```python
from build123d import *

# Parameters (mm, degrees)
F1_DEPTH = 33.02
F0_R     = 2.6264362
F0_R_2   = 2.6264304873
F2_DEPTH = 38.1


with BuildPart() as f1:
    # F0 (on Front) → F1 (new body, symmetric)
    with BuildSketch(Plane.XZ):
        with BuildLine():
            add(Edge.make_bspline(
                [(-31.4454593495, -10.5763216779), (-18.4102778878, -14.3703602753), (-20.5599198365, -22.9724258326), (-15.1177148521, -29.1741350755)],
                knots=[0, 0, 0, 0, 24.7482101079, 24.7482101079, 24.7482101079, 24.7482101079], degree=3))
            ThreePointArc((-31.4454593495, -10.5763216779), (-36.4175873656, -8.3966690551), (-39.6507896865, -4.035551616))
            Line((-39.6507896865, -4.035551616), (-31.297441197, -25.0651440107))
            ThreePointArc((-31.297441197, -25.0651440107), (-29.241828265, -28.1482147194), (-26.1079207685, -30.1254585901))
            Line((-26.1079207685, -30.1254585901), (-3.0730358258, -38.6095386283))
            ThreePointArc((-3.0730358258, -38.6095386283), (-1.5607510796, -39.0193916461), (0, -39.1573797531))
            Line((0, -39.1573797531), (0, -37.687844526))
            ThreePointArc((0, -37.687844526), (-8.6750871891, -35.4130686309), (-15.1177148521, -29.1741350755))
        make_face()
        with BuildLine():
            ThreePointArc((33.6601813113, -9.9752325779), (32.9890386835, -10.2112882492), (32.3035305265, -10.4016386456))
            add(Edge.make_bspline(
                [(32.3035305265, -10.4016386456), (18.5081026821, -15.0106381958), (21.1109032546, -22.9743855244), (15.1177148521, -29.1741350755)],
                knots=[0.8170048254, 0.8170048254, 0.8170048254, 0.8170048254, 26.6912142755, 26.6912142755, 26.6912142755, 26.6912142755], degree=3))
            ThreePointArc((15.1177148521, -29.1741350755), (8.6750871891, -35.4130686309), (0, -37.687844526))
            Line((0, -37.687844526), (0, -39.1573797531))
            ThreePointArc((0, -39.1573797531), (1.5607053421, -39.0192220029), (3.0729166956, -38.6092152337))
            Line((3.0729166956, -38.6092152337), (27.1625130087, -29.7337906358))
            ThreePointArc((27.1625130087, -29.7337906358), (30.2961519286, -27.7562759529), (32.3514385124, -24.6730869774))
            Line((32.3514385124, -24.6730869774), (39.6400981385, -4.0318907199))
            ThreePointArc((39.6400981385, -4.0318907199), (37.2687025045, -7.6259310267), (33.6601813113, -9.9752325779))
        make_face()
    extrude(amount=F1_DEPTH, both=True)

    # F0 (on Front) → F2 (join, symmetric)
    with BuildSketch(Plane.XZ):
        with BuildLine():
            ThreePointArc((-31.4454593495, -10.5763216779), (-22.9558140486, -8.155960982), (-19.2675045322, -0.1354500166))
            ThreePointArc((-19.2675045322, -0.1354500166), (-22.3620278457, 7.3351409283), (-29.8327647689, 10.4293118073))
            ThreePointArc((-29.8327647689, 10.4293118073), (-38.5736258357, 5.7977470387), (-39.6507896865, -4.035551616))
            ThreePointArc((-39.6507896865, -4.035551616), (-36.4175873656, -8.3966690551), (-31.4454593495, -10.5763216779))
        make_face()
        with Locations((-27.8002675623, -4.0318907199)):
            Circle(F0_R, mode=Mode.SUBTRACT)
        with BuildLine():
            ThreePointArc((-29.8327647689, 10.4293118073), (-22.3620278457, 7.3351409283), (-19.2675045322, -0.1354500166))
            Line((-19.2675045322, -0.1354500166), (0, -0.1354500166))
            Line((0, -0.1354500166), (0, 10.4307191917))
            Line((0, 10.4307191917), (-29.8327647689, 10.4293118073))
        make_face()
        with BuildLine():
            Line((0, 10.4307191917), (0, -0.1354500166))
            Line((0, -0.1354500166), (19.2564770783, -0.1354500166))
            ThreePointArc((19.2564770783, -0.1354500166), (22.3496527134, 7.3366076469), (29.8207401381, 10.4321260089))
            Line((29.8207401381, 10.4321260089), (0, 10.4307191917))
        make_face()
        with BuildLine():
            ThreePointArc((29.8207401381, 10.4321260089), (22.3496527134, 7.3366076469), (19.2564770783, -0.1354500166))
            Line((19.2564770783, -0.1354500166), (40.386, -0.1354500166))
            ThreePointArc((40.386, -0.1354500166), (40.3860002811, -0.1340429158), (40.3860003748, -0.132635815))
            ThreePointArc((40.3860003748, -0.132635815), (37.2914770613, 7.3379551299), (29.8207401381, 10.4321260089))
        make_face()
        with BuildLine():
            Line((40.386, -0.1354500166), (19.2564770783, -0.1354500166))
            ThreePointArc((19.2564770783, -0.1354500166), (23.2882273315, -8.4352834172), (32.3035305265, -10.4016386456))
            add(Edge.make_bspline(
                [(33.6601813113, -9.9752325779), (33.1910900089, -10.1139156622), (32.7391353761, -10.2561047355), (32.3035305265, -10.4016386456)],
                knots=[0, 0, 0, 0, 0.8170048254, 0.8170048254, 0.8170048254, 0.8170048254], degree=3))
            ThreePointArc((33.6601813113, -9.9752325779), (37.2687025045, -7.6259310267), (39.6400981385, -4.0318907199))
            ThreePointArc((39.6400981385, -4.0318907199), (40.1975849298, -2.1189963626), (40.386, -0.1354500166))
        make_face()
        with Locations((29.3497324377, -4.0318907199)):
            Circle(F0_R_2, mode=Mode.SUBTRACT)
        with BuildLine():
            Line((19.2564770783, -0.1354500166), (0, -0.1354500166))
            Line((0, -0.1354500166), (0, -2.329749126))
            ThreePointArc((0, -2.329749126), (12.5009745136, -7.5078223124), (17.6790477, -20.008796826))
            ThreePointArc((17.6790477, -20.008796826), (17.0266780313, -24.7670488997), (15.1177148521, -29.1741350755))
            add(Edge.make_bspline(
                [(32.3035305265, -10.4016386456), (18.5081026821, -15.0106381958), (21.1109032546, -22.9743855244), (15.1177148521, -29.1741350755)],
                knots=[0.8170048254, 0.8170048254, 0.8170048254, 0.8170048254, 26.6912142755, 26.6912142755, 26.6912142755, 26.6912142755], degree=3))
            ThreePointArc((32.3035305265, -10.4016386456), (23.2882273315, -8.4352834172), (19.2564770783, -0.1354500166))
        make_face()
        with BuildLine():
            ThreePointArc((17.6790477, -20.008796826), (12.5009745136, -7.5078223124), (0, -2.329749126))
            Line((0, -2.329749126), (0, -5.484860926))
            ThreePointArc((0, -5.484860926), (10.2699735644, -9.7388232616), (14.5239359, -20.008796826))
            ThreePointArc((14.5239359, -20.008796826), (10.2699735644, -30.2787703904), (0, -34.532732726))
            Line((0, -34.532732726), (0, -37.687844526))
            ThreePointArc((0, -37.687844526), (8.6750871891, -35.4130686309), (15.1177148521, -29.1741350755))
            ThreePointArc((15.1177148521, -29.1741350755), (17.0266780313, -24.7670488997), (17.6790477, -20.008796826))
        make_face()
        with BuildLine():
            Line((0, -0.1354500166), (-19.2675045322, -0.1354500166))
            ThreePointArc((-19.2675045322, -0.1354500166), (-22.9558140486, -8.155960982), (-31.4454593495, -10.5763216779))
            add(Edge.make_bspline(
                [(-31.4454593495, -10.5763216779), (-18.4102778878, -14.3703602753), (-20.5599198365, -22.9724258326), (-15.1177148521, -29.1741350755)],
                knots=[0, 0, 0, 0, 24.7482101079, 24.7482101079, 24.7482101079, 24.7482101079], degree=3))
            ThreePointArc((-15.1177148521, -29.1741350755), (-15.4042718049, -11.3337096369), (0, -2.329749126))
            Line((0, -2.329749126), (0, -0.1354500166))
        make_face()
        with BuildLine():
            Line((0, -5.484860926), (0, -2.329749126))
            ThreePointArc((0, -2.329749126), (-15.4042718049, -11.3337096369), (-15.1177148521, -29.1741350755))
            ThreePointArc((-15.1177148521, -29.1741350755), (-8.6750871891, -35.4130686309), (0, -37.687844526))
            Line((0, -37.687844526), (0, -34.532732726))
            ThreePointArc((0, -34.532732726), (-14.5239359, -20.008796826), (0, -5.484860926))
        make_face()
        with BuildLine():
            Line((0, -34.532732726), (0, -5.484860926))
            ThreePointArc((0, -5.484860926), (-14.5239359, -20.008796826), (0, -34.532732726))
        make_face()
        with BuildLine():
            ThreePointArc((14.5239359, -20.008796826), (10.2699735644, -9.7388232616), (0, -5.484860926))
            Line((0, -5.484860926), (0, -34.532732726))
            ThreePointArc((0, -34.532732726), (10.2699735644, -30.2787703904), (14.5239359, -20.008796826))
        make_face()
    extrude(amount=F2_DEPTH, both=True)


solid = f1.part
```
Geometry: final body of the model. Coordinates: model frame, mm. A direction names the side the tool comes from. Coordinates: 2 decimals unless noted, no trailing zeros. Order: outer loops, then holes, each group sorted by start corner. A loop starts at its lowest first (then second) coordinate and runs counter-clockwise, first axis right, second up. Notation, with made-up numbers: (-8, 9) - (36, 9) arc R36 cw to (36, 48) - close; hole circle Ø11 at (30, -24). An arc over 180 degrees is marked (long way). Return JSON: item names as keys, results as strings. Group by question number.
1. Cut plane B-B (z = -35.5). Output: boundary loops of the cut face in (x, y), plus the area to 3 significant figures.
2. Material intervals for line 1 along X through (y, z) = (-21.5, -3.5); line 2 along Z through (x, y) = (27, 8); line 3 along Y through (x, z) = (27.5, -23), sorted ascending. Write a range as [from, to].
3. Cut plane A-A (y = -3). Count the separate pieces of the cut face and the enclosed holes in it, plus the area to 3 significant figures.
4. Cut plane C-C (z = 6.5). Output: boundary loops of the cut face in (x, y), plus the area to 3 significant figures.
5. Pin query (flat end, axial travel): pin 1 (10 mm diameter, centred on x = -18, y = 16, fed in from +Z); pin 2 (2 mm diameter, centred on y = -10, z = -25.5, fed in from -X); pin 3 (5 mm diameter, centred on y = -25.5, z = -7, fed in from +X). Return the tip coordinate at first contact, or that it passes through.
6. Set-up query: faces 1 (the face through (9, 33.02, -36)), 2 (the face through (9, -33.02, -36)), 3 (the face through (39.776, -0.533, -3.672)). Return all of +Z, -Z, +X, -X, +Y, -Y with unobstructed straight access to the full face (end or side cutting, diameter ignored); none if empty.
Resolved:
{
 "1": {"outline": "(-11.52, -33.02) - (-8.52, -33.02) - (-8.52, -38.1) - (8.52, -38.1) - (8.52, -33.02) - (11.51, -33.02) - (11.51, 33.02) - (8.52, 33.02) - (8.52, 38.1) - (-8.52, 38.1) - (-8.52, 33.02) - (-11.52, 33.02) - close", "area": "1,690 mm²"},
 "2": {"line 1": "x = [-39.85, -30.37], [-25.23, 26.78], [31.92, 39.83]", "line 2": "z = [-29.79, -5.21], [-2.86, 10.43]", "line 3": "y = [-33.02, 33.02]"},
 "3": {"separate pieces": "1", "enclosed holes": "3", "area": "3,130 mm²"},
 "4": {"outline": "(-38.05, -38.1) - (38.04, -38.1) - (38.04, 38.1) - (-38.05, 38.1) - close", "area": "5,800 mm²"},
 "5": {"pin 1": "stops at z = 10.43", "pin 2": "stops at x = -31.52", "pin 3": "stops at x = 39.47"},
 "6": {"face 1": "-Z, +Y", "face 2": "-Z, -Y", "face 3": "-Z, +X"}
}
